For this review, take the finished solid that the model builds, in its own axes (mm). A direction names the side the tool comes from. Give positions to 0.01 mm unless a question says otherwise; leave off trailing zeros. Write each loop counter-clockwise with the first axis right and the second up, starting at its lowest first coordinate (ties: lowest second). Pieces come first, ordered by that corner, then holes.
Q1. Machinability: for faces 1 (the cylindrical face through (-42.64, -4.56, -2.9)), 2 (the flat face through (60, 1, 27.7)), 3 (the cylindrical face through (-45.36, 6.4, -4.52)), 4 (the cylindrical face through (62.817, 2.621, 21.922)), 5 (the flat face through (-37, -4, 3)), which of the approach directions +Z, -Z, +X, -X, +Y, -Y give a long, thin tool a straight path to every point of the face, cutting with its end or side? Answer none if there is none.
Q2. For line 1 (X direction, y = -3, z = 4.5); line 2 (X direction, y = 3.5, z = 10); line 3 (X direction, y = -4.5, z = 27.5), list the stretches that pass through material, from the lowest coordinate up.
Q3. Mouldability with a two-part tool opening along Z and no side actions: class faces 6 (the cylindrical face through (42.6, -4.56, -2.86)), 7 (the flat face through (-24.39, -6.89, 4.28)), 8 (the flat face through (-70, 3, 4)) as released by +Z, released by -Z, zero draft, split by the parting line, or undercut.
Q4. We need section C-C (x = 49.8). Write out the cut boundary in (y, z), then the cut area to 3 significant figures.
Q5. We need section D-D (x = -2.5). Write out the cut boundary in (y, z).
Q6. We need section B-B (z = 11.5). Write out the cut boundary in (x, y).
Q7. We need section A-A (x = 73). Write out the cut boundary in (y, z), then the cut area to 3 significant figures.
Q8. Insertion check: P1, Ø3, axis at x = -25, y = -5.5, coming from the -Z side; P2, Ø4.5, axis at y = -3.5, z = 26.5, coming from the +X side; P3, Ø4, axis at x = -26, y = -6, coming from the +Z side. Each pin has a flat end and moves straight along its axis. Give the tip position at first contact, or say it passes through.
```python
from build123d import *

# Parameters (mm, degrees)
F2_DEPTH  = 9
F3_DEPTH  = 10
F4_R      = 1.75
F5_DEPTH  = 158.2
F4_R_2    = 3.25
F6_DEPTH  = 2.4
F7_R      = 3.25
F8_DEPTH  = 2.4
F9_R      = 3.4
F9_R_2    = 1.75
F10_DEPTH = 3
F11_DEPTH = 25
F12_W     = 100
F12_H     = 9
F13_DEPTH = 1.1
F14_W     = 19
F14_H     = 10
F15_DEPTH = 16
F16_SIZE  = 5
F17_W     = 19
F17_H     = 10
F18_DEPTH = 16
F19_SIZE  = 5
F20_R     = 3.15
F21_DEPTH = 25
F22_R     = 0.4
F23_W     = 87
F23_H     = 9
F24_DEPTH = 4
F25_R     = 3
F26_W     = 33
F26_H     = 9
F26_R     = 1.6
F27_DEPTH = 18
F28_DEPTH = 30
F30_DEPTH = 2.6
F31_R     = 1.6
F32_DEPTH = 12.5
F34_DEPTH = 2.6
F35_W     = 5.5
F35_H     = 2.6
F36_DEPTH = 3.7
F37_R     = 0.5


with BuildPart() as f2:
    # F1 (on face) → F2 (new body)
    with BuildSketch(Plane.XZ):
        Polygon((-55, 27.7), (-64, 27.7), (-64, -6), (0, -6), (64, -6), (64, 27.7), (55, 27.7), (55, 31.9), (0, 31.9), (-55, 31.9), align=None)
    extrude(amount=F2_DEPTH)

    # F0 (on Front) → F3 (join)
    with BuildSketch(Plane.XZ):
        with BuildLine():
            Line((-57.5, 27.7), (-64, 27.7))
            Line((-64, 27.7), (-64, -6))
            Line((-64, -6), (-43.5, -6))
            Line((-43.5, -6), (-43.5, 0))
            Line((-43.5, 0), (-55, 0))
            ThreePointArc((-55, 0), (-55.3535533906, -0.1464466094), (-55.5, -0.5))
            Line((-55.5, -0.5), (-55.5, -1.8))
            Line((-55.5, -1.8), (-59, -1.8))
            Line((-59, -1.8), (-59, 6.2))
            Line((-59, 6.2), (-54.7, 6.2))
            ThreePointArc((-54.7, 6.2), (-54.3464466094, 6.3464466094), (-54.2, 6.7))
            Line((-54.2, 6.7), (-54.2, 13.2))
            ThreePointArc((-54.2, 13.2), (-54.3464466094, 13.5535533906), (-54.7, 13.7))
            Line((-54.7, 13.7), (-59, 13.7))
            Line((-59, 13.7), (-59, 20.2))
            Line((-59, 20.2), (-57.5, 20.2))
            ThreePointArc((-57.5, 20.2), (-57.1464466094, 20.3464466094), (-57, 20.7))
            Line((-57, 20.7), (-57, 27.2))
            ThreePointArc((-57, 27.2), (-57.1464466094, 27.5535533906), (-57.5, 27.7))
        make_face()
        with BuildLine():
            Line((43.5, -6), (64, -6))
            Line((64, -6), (64, 27.7))
            Line((64, 27.7), (57.5, 27.7))
            ThreePointArc((57.5, 27.7), (57.1464466094, 27.5535533906), (57, 27.2))
            Line((57, 27.2), (57, 20.7))
            ThreePointArc((57, 20.7), (57.1464466094, 20.3464466094), (57.5, 20.2))
            Line((57.5, 20.2), (59, 20.2))
            Line((59, 20.2), (59, 13.7))
            Line((59, 13.7), (54.7, 13.7))
            ThreePointArc((54.7, 13.7), (54.3464466094, 13.5535533906), (54.2, 13.2))
            Line((54.2, 13.2), (54.2, 6.7))
            ThreePointArc((54.2, 6.7), (54.3464466094, 6.3464466094), (54.7, 6.2))
            Line((54.7, 6.2), (59, 6.2))
            Line((59, 6.2), (59, -1.8))
            Line((59, -1.8), (55.5, -1.8))
            Line((55.5, -1.8), (55.5, -0.5))
            ThreePointArc((55.5, -0.5), (55.3535533906, -0.1464466094), (55, 0))
            Line((55, 0), (43.5, 0))
            Line((43.5, 0), (43.5, -6))
        make_face()
    extrude(amount=-F3_DEPTH)

    # F4 (on face) → F5 (cut)
    with BuildSketch(Plane(origin=(-64, 0, 0), x_dir=(0, -1, 0), z_dir=(-1, 0, 0))):
        with Locations((-5.2, 23.9)):
            Circle(F4_R)
    extrude(amount=-F5_DEPTH, mode=Mode.SUBTRACT)

    # F4 (on face) → F6 (cut)
    with BuildSketch(Plane(origin=(-64, 0, 0), x_dir=(0, -1, 0), z_dir=(-1, 0, 0))):
        with Locations((-5.2, 23.9)):
            Circle(F4_R_2)
        with Locations((-5.2, 23.9)):
            Circle(F4_R, mode=Mode.SUBTRACT)
    extrude(amount=-F6_DEPTH, mode=Mode.SUBTRACT)

    # F7 (on face) → F8 (cut)
    with BuildSketch(Plane.YZ.offset(64)):
        with Locations((5.2, 23.9)):
            Circle(F7_R)
    extrude(amount=-F8_DEPTH, mode=Mode.SUBTRACT)

    # F9 (on face) → F10 (cut)
    with BuildSketch(Plane(origin=(0, 0, -6), x_dir=(1, 0, 0), z_dir=(0, 0, -1))):
        with Locations((49.8, -5.1)):
            Circle(F9_R)
        with Locations((49.8, -5.1)):
            Circle(F9_R_2, mode=Mode.SUBTRACT)
        with Locations((-48.5, -5.1)):
            Circle(F9_R)
        with Locations((-48.5, -5.1)):
            Circle(F9_R_2, mode=Mode.SUBTRACT)
        with Locations((49.8, -5.1)):
            Circle(F9_R_2)
    extrude(amount=-F10_DEPTH, mode=Mode.SUBTRACT)

    # F9 (on face) → F11 (cut)
    with BuildSketch(Plane(origin=(0, 0, -6), x_dir=(1, 0, 0), z_dir=(0, 0, -1))):
        with Locations((49.8, -5.1)):
            Circle(F9_R_2)
        with Locations((-48.5, -5.1)):
            Circle(F9_R_2)
    extrude(amount=-F11_DEPTH, mode=Mode.SUBTRACT)

    # F12 (on face) → F13 (join)
    with BuildSketch(Plane.XY.offset(31.9)):
        with Locations((-5, -4.5)):
            Rectangle(F12_W, F12_H)
    extrude(amount=F13_DEPTH)

    # F14 (on face) → F15 (join)
    with BuildSketch(Plane(origin=(-64, 0, 0), x_dir=(0, -1, 0), z_dir=(-1, 0, 0))):
        with Locations((-0.5, -1)):
            Rectangle(F14_W, F14_H)
    extrude(amount=F15_DEPTH)

    # F16
    f16_edges = [f2.edges().sort_by_distance(p)[0] for p in [
        (-80, -9, -1),
        (-80, 10, -1),
    ]]
    chamfer(f16_edges, length=F16_SIZE)

    # F17 (on face) → F18 (join)
    with BuildSketch(Plane.YZ.offset(64)):
        with Locations((0.5, -1)):
            Rectangle(F17_W, F17_H)
    extrude(amount=F18_DEPTH)

    # F19
    f19_edges = [f2.edges().sort_by_distance(p)[0] for p in [
        (80, 10, -1),
        (80, -9, -1),
    ]]
    chamfer(f19_edges, length=F19_SIZE)

    # F20 (on face) → F21 (cut)
    with BuildSketch(Plane(origin=(0, 0, -6), x_dir=(1, 0, 0), z_dir=(0, 0, -1))):
        with Locations((-73, -0.5)):
            Circle(F20_R)
        with Locations((73, -0.5)):
            Circle(F20_R)
    extrude(amount=-F21_DEPTH, mode=Mode.SUBTRACT)

    # F22
    f22_edges = [f2.edges().sort_by_distance(p)[0] for p in [
        (64, 0.5, 27.7),
        (45, -4.5, 33),
        (-64, 0.5, 27.7),
        (-55, -4.5, 27.7),
        (-55, -4.5, 33),
        (-64, 0.5, 4),
        (64, 0.5, 4),
    ]]
    fillet(f22_edges, radius=F22_R)

    # F23 (on face) → F24 (cut)
    with BuildSketch(Plane(origin=(0, 0, -6), x_dir=(1, 0, 0), z_dir=(0, 0, -1))):
        with Locations((0, 4.5)):
            Rectangle(F23_W, F23_H)
    extrude(amount=-F24_DEPTH, mode=Mode.SUBTRACT)

    # F25
    f25_edges = [f2.edges().sort_by_distance(p)[0] for p in [
        (-43.5, -4.5, -2),
        (43.5, -4.5, -2),
    ]]
    fillet(f25_edges, radius=F25_R)

    # F26 (on face) → F27 (cut)
    with BuildSketch(Plane.XY.offset(33)):
        with Locations((-31.5, -4.5)):
            Rectangle(F26_W, F26_H)
        with Locations((-37.25, -4.5)):
            Circle(F26_R, mode=Mode.SUBTRACT)
        with Locations((-25.75, -4.5)):
            Circle(F26_R, mode=Mode.SUBTRACT)
    extrude(amount=-F27_DEPTH, mode=Mode.SUBTRACT)

    # F26 (on face) → F28 (cut)
    with BuildSketch(Plane.XY.offset(33)):
        with Locations((-37.25, -4.5)):
            Circle(F26_R)
        with Locations((-25.75, -4.5)):
            Circle(F26_R)
    extrude(amount=-F28_DEPTH, mode=Mode.SUBTRACT)

    # F29 (on face) → F30 (cut)
    with BuildSketch(Plane.XY.offset(3)):
        Polygon((-28.5, -2.9122867597), (-28.5, -6.0877132403), (-25.75, -7.6754264805), (-23, -6.0877132403), (-23, -2.9122867597), (-25.75, -1.3245735195), align=None)
        Polygon((-40, -2.9122867597), (-40, -6.0877132403), (-37.25, -7.6754264805), (-34.5, -6.0877132403), (-34.5, -2.9122867597), (-37.25, -1.3245735195), align=None)
    extrude(amount=F30_DEPTH, mode=Mode.SUBTRACT)

    # F31 (on face) → F32 (cut)
    with BuildSketch(Plane.XY.offset(33)):
        with Locations((-8, -4.5)):
            Circle(F31_R)
        with Locations((8, -4.5)):
            Circle(F31_R)
    extrude(amount=-F32_DEPTH, mode=Mode.SUBTRACT)

    # F33 (on face) → F34 (cut)
    with BuildSketch(Plane.XY.offset(20.5)):
        Polygon((-5.25, -6.0877132403), (-5.25, -2.9122867597), (-8, -1.3245735195), (-10.75, -2.9122867597), (-10.75, -6.0877132403), (-8, -7.6754264805), align=None)
        Polygon((10.75, -6.0877132403), (10.75, -2.9122867597), (8, -1.3245735195), (5.25, -2.9122867597), (5.25, -6.0877132403), (8, -7.6754264805), align=None)
    extrude(amount=F34_DEPTH, mode=Mode.SUBTRACT)

    # F35 (on face) → F36 (cut)
    with BuildSketch(Plane(origin=(0, 0, 0), x_dir=(-1, 0, 0), z_dir=(0, 1, 0))):
        with Locations((-8, 21.8)):
            Rectangle(F35_W, F35_H)
        with Locations((8, 21.8)):
            Rectangle(F35_W, F35_H)
        with Locations((25.75, 4.3)):
            Rectangle(F35_W, F35_H)
        with Locations((37.25, 4.3)):
            Rectangle(F35_W, F35_H)
    extrude(amount=-F36_DEPTH, mode=Mode.SUBTRACT)

    # F37
    f37_edges = [f2.edges().sort_by_distance(p)[0] for p in [
        (-15, -4.5, 33),
        (-15, -4.5, 15),
        (-48, -4.5, 15),
        (-48, -4.5, 33),
    ]]
    fillet(f37_edges, radius=F37_R)


solid = f2.part
```
Computed:
1. face 1: -Z, +Y, -Y
1. face 2: +Z, +X, +Y, -Y
1. face 3: -Z
1. face 4: +X
1. face 5: +Y
2. line 1: x = -64 to -40, -34.5 to -28.5, -23 to 64
2. line 2: x = -64 to -54.2, 54.2 to 64
2. line 3: x = -63.95 to -48, -15 to -9.6, -6.4 to 6.4, 9.6 to 63.95
3. face 6: released by -Z
3. face 7: undercut
3. face 8: released by +Z
4. outline: (-9, -6) - (1.7, -6) - (1.7, -3) - (3.35, -3) - (3.35, 0) - (0, 0) - (0, 31.9) - (-9, 31.9) - close; (6.85, -3) - (8.5, -3) - (8.5, -6) - (10, -6) - (10, 0) - (6.85, 0) - close
4. area: 370 mm2
5. outline: (-9, -2) - (0, -2) - (0, 33) - (-9, 33) - close
6. outline: (-64, -9) - (64, -9) - (64, 10) - (54.2, 10) - (54.2, 0) - (-54.2, 0) - (-54.2, 10) - (-64, 10) - close; hole circle Ø3.2 at (-37.25, -4.5); hole circle Ø3.2 at (-25.75, -4.5)
7. outline: (-9, -6) - (-2.65, -6) - (-2.65, 4) - (-9, 4) - close; (3.65, -6) - (10, -6) - (10, 4) - (3.65, 4) - close
7. area: 127 mm2
8. P1: stops at z = -2
8. P2: stops at x = 64
8. P3: stops at z = 15
